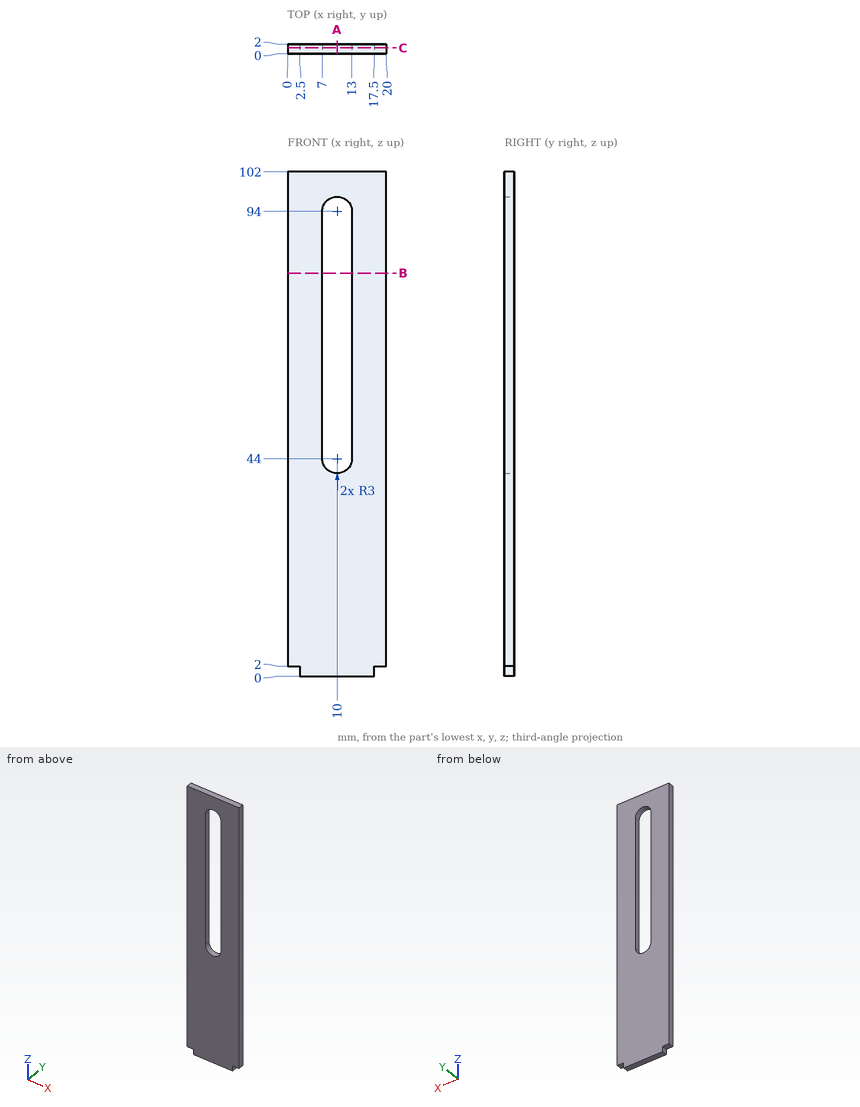
Input: dimensioned drawing with shaded views. Units: mm. Origin: part minimum x, y, z. Give positions to 0.01 mm unless a question says otherwise; leave off trailing zeros. Loops run counter-clockwise (first coordinate to the right, second up) from the corner with the lowest first, then second, coordinate; pieces in that order, holes last. Notation, with made-up numbers: M 22,38.5 L 37,38.5 A16 cw 37,61.5 Z; hole C -15.75,52 d3. An arc over 180 degrees is marked long. Put each result on its own line as item: value. Start each with the question number.
1) Cut plane B-B (z = 81.5). Output: boundary loops of the cut face in (x, y).
2) Contact query for flat-ended pins moving along their axis: pin 1 (0.6 mm diameter, centred on y = 0.5, z = 1, fed in from +X); pin 2 (0.6 mm diameter, centred on y = 1, z = 0.5, fed in from -X). Output: stop coordinate, or through.
3) Cut plane C-C (y = 1.2). Output: boundary loops of the cut face in (x, z), then the cut area to 3 significant figures.
4) Ray query, line 1 along X through (y, z) = (0.1, 54.5); line 2 along Z through (x, y) = (8.5, 1.15); line 3 along Z through (x, y) = (7.5, 0.2). Return the intervals inside material, ascending.
5) Cut plane A-A (x = 10). Output: boundary loops of the cut face in (y, z).
Verdict:
1. outline: M 0,0 L 7,0 L 7,2 L 0,2 Z; M 13,0 L 20,0 L 20,2 L 13,2 Z
2. pin 1: x = 17.5
2. pin 2: x = 2.5
3. outline: M 0,2 L 2.5,2 L 2.5,0 L 17.5,0 L 17.5,2 L 20,2 L 20,102 L 0,102 Z; hole M 7,44 A3 ccw 13,44 L 13,94 A3 ccw 7,94 Z
3. area: 1,700 mm2
4. line 1: 0 to 7, 13 to 20
4. line 2: 0 to 41.4, 96.6 to 102
4. line 3: 0 to 42.34, 95.66 to 102
5. outline: M 0,0 L 2,0 L 2,41 L 0,41 Z; M 0,97 L 2,97 L 2,102 L 0,102 Z
